Could you check a few things on this model? Use its own coordinates, in mm. A direction names the side the tool comes from. Give positions to 0.01 mm unless a question says otherwise; leave off trailing zeros. Loops run counter-clockwise (first coordinate to the right, second up) from the corner with the lowest first, then second, coordinate; pieces in that order, holes last. Notation, with made-up numbers: (54.25, 53) - (101.25, 53) arc R11 cw to (101.25, 73) - close; hole circle Ø9 at (-15.5, 30). An arc over 180 degrees is marked (long way). Write each question's results on one line, items separated by ' | '. Start each with the question number.
(1) If we mould it in two halves opening along Y, with no side actions, what happens to faces 1 (the face through (45, -58, 24)), 2 (the face through (45, -47, 47.4)), 3 (the face through (45.343, -67.231, 43.636))? For each: released by +Y, released by -Y, zero draft, split by the parting line, or undercut.
(2) Suppose I cut it at D-D (y = -61.5). Please give me the cut outline in (x, z).
(3) I need wall thicknesses on line 1 (Y direction, x = 39.5, z = 29); line 2 (Z direction, x = 52, y = -56.5); line 3 (Y direction, x = 24.5, z = 13). Which ranges of each line are inside material? Lowest first, please.
(4) Suppose I cut it at C-C (x = 39). Please give me the cut outline in (y, z).
(5) Suppose I cut it at A-A (z = 16.5). Please give me the cut outline in (x, y), and give its area (3 significant figures).
(6) Suppose I cut it at B-B (y = -48). Please give me the cut outline in (x, z).
(7) On a 3-axis mill with a long thin cutter (end or side, diameter ignored), from which of +Z, -Z, +X, -X, +Y, -Y can I reach the whole of each face in a straight line? I mean faces 4 (the face through (45, -23.8, 24)), 5 (the face through (45, -47, 13.2)). Say none if no direction works.
Autodesk Inventor part; units mm, degrees
ref_plane "YZ Plane" through (0, 0, 0) normal (1, 0, 0) x (0, 1, 0)
ref_plane "XZ Plane" through (0, 0, 0) normal (0, 1, 0) x (-1, 0, 0)
ref_plane "XY Plane" through (0, 0, 0) normal (0, 0, 1) x (1, 0, 0)
sketch "Sketch1" plane through (0, 0, 0) normal (0, 0, 1) x (1, 0, 0)
  point P0 (0, 0)
sketch "LAYER1" plane through (0, 0, 0) normal (0, 0, 1) x (1, 0, 0)
  line L0 (70, 20.5) -> (90, 20.5)
  line L1 (90, 20.5) -> (90, 57.5)
  line L2 (90, 57.5) -> (0, 57.5)
  line L3 (0, 57.5) -> (0, -57.5)
  line L4 (0, -57.5) -> (90, -57.5)
  line L5 (90, -57.5) -> (90, -20.5)
  line L6 (90, -20.5) -> (70, -20.5)
  line L7 (70, -20.5) -> (70, -37.5)
  line L8 (70, -37.5) -> (20, -37.5)
  line L9 (20, -37.5) -> (20, 37.5)
  line L10 (20, 37.5) -> (70, 37.5)
  line L11 (70, 37.5) -> (70, 20.5)
sketch "LAYER2" plane through (0, 0, 0) normal (0, 0, 1) x (1, 0, 0)
  line L0 (20.1, -20) -> (110.1, -20)
  line L1 (110.1, -20) -> (110.1, 20)
  line L2 (110.1, 20) -> (20.1, 20)
  line L3 (20.1, 20) -> (20.1, -20)
sketch "LAYER3" plane through (0, 0, 0) normal (0, 0, 1) x (1, 0, 0)
  line L0 (20.5, -71.2) -> (69.5, -71.2)
  line L1 (69.5, -71.2) -> (69.5, -58)
  line L2 (69.5, -58) -> (20.5, -58)
  line L3 (20.5, -58) -> (20.5, -71.2)
sketch "LAYER4" plane through (0, 0, 0) normal (0, 0, 1) x (1, 0, 0)
  line L0 (20.5, -23.8) -> (69.5, -23.8)
  line L1 (69.5, -23.8) -> (69.5, -37)
  line L2 (69.5, -37) -> (20.5, -37)
  line L3 (20.5, -37) -> (20.5, -23.8)
sketch "LAYER5" plane through (0, 0, 0) normal (0, 0, 1) x (1, 0, 0)
  line L0 (20.5, 23.8) -> (69.5, 23.8)
  line L1 (69.5, 23.8) -> (69.5, 37)
  line L2 (69.5, 37) -> (20.5, 37)
  line L3 (20.5, 37) -> (20.5, 23.8)
sketch "LAYER6" plane through (0, 0, 0) normal (0, 0, 1) x (1, 0, 0)
  line L0 (20.5, 71.2) -> (69.5, 71.2)
  line L1 (69.5, 71.2) -> (69.5, 58)
  line L2 (69.5, 58) -> (20.5, 58)
  line L3 (20.5, 58) -> (20.5, 71.2)
extrude "Extrusion3" add sketch "LAYER3" along normal blind 47.4
extrude "Extrusion4" add sketch "LAYER4" along normal blind 47.4
sketch "Sketch9" plane through (20.5, -37, 0) normal (-1, 0, 0) x (0, 0, 1)
  line L0 (0, 0) -> (47.4, 0)
  line L1 (0, -21) -> (47.4, -21)
  line L2 (47.4, 0) -> (47.4, -21)
  line L3 (0, 0) -> (0, -21)
  line L4 (13.2, 0) -> (13.2, -21)
  line L5 (34.2, 0) -> (34.2, -21)
  point P0 (0, 37)
  dimension "d12" = 13.2
  dimension "d13" = 13.2
extrude "Extrusion6" add sketch "Sketch9" against normal up to surface (49 mm away) contours L0 L4 L1 L3 | L0 L2 L1 L5
fillet "Fillet1" radius 13.2 4 edges at (45, -23.8, 47.4) (45, -71.2, 47.4) (45, -71.2, 0) (45, -23.8, 0)
properties part number "Winding"
Output values:
1) face 1: undercut | face 2: zero draft | face 3: released by -Y
2) outline: (20.5, 0.47) - (69.5, 0.47) - (69.5, 46.93) - (20.5, 46.93) - close
3) line 1: -71.2 to -58, -37 to -23.8 | line 2: 0 to 13.2, 34.2 to 47.4 | line 3: -71.2 to -23.8
4) outline: (-71.2, 13.2) arc R13.2 ccw to (-58, 0) - (-37, 0) arc R13.2 ccw to (-23.8, 13.2) - (-23.8, 34.2) arc R13.2 ccw to (-37, 47.4) - (-58, 47.4) arc R13.2 ccw to (-71.2, 34.2) - close; hole (-58, 13.2) - (-37, 13.2) - (-37, 34.2) - (-58, 34.2) - close
5) outline: (20.5, -71.2) - (69.5, -71.2) - (69.5, -58) - (20.5, -58) - close; (20.5, -37) - (69.5, -37) - (69.5, -23.8) - (20.5, -23.8) - close | area: 1,290 mm2
6) outline: (20.5, 0) - (69.5, 0) - (69.5, 13.2) - (20.5, 13.2) - close; (20.5, 34.2) - (69.5, 34.2) - (69.5, 47.4) - (20.5, 47.4) - close
7) face 4: +Z, -Z, +X, -X, +Y | face 5: +X, -X
